from build123d import *

# Parameters (mm, degrees)
EXTRUDE_1_DEPTH      = 4
EXTRUDE_1_2_DEPTH    = 4
EXTRUDE_1_3_DEPTH    = 4
SKETCH_2_W           = 7
SKETCH_2_H           = 5
EXTRUDE_2_DEPTH      = 0.6
SKETCH_3_W           = 4.85
SKETCH_3_H           = 1.2
EXTRUDE_3_DEPTH      = 0.6
SKETCH_4_W           = 1
SKETCH_4_H           = 13.65
EXTRUDE_4_DEPTH      = 0.6
FILLET_1_R           = 0.5
FILLET_2_R           = 0.3
SKETCH_5_W           = 1.1
SKETCH_5_H           = 0.6
EXTRUDE_5_DEPTH      = 2
EXTRUDE_5_DEPTH_BACK = 18


with BuildPart() as part:
    # Sketch 1 → Extrude 1 (new body)
    with BuildSketch(Plane(origin=(0, 0, 0), x_dir=(1, 0, 0), z_dir=(0, 1, 0))):
        with BuildLine():
            Line((-2.2, 1.245389122), (2.2, 1.245389122))
            ThreePointArc((2.2, 1.245389122), (2.694974747, 1.040363869), (2.9, 0.545389122))
            Line((2.9, 0.545389122), (2.9, -1.454610878))
            ThreePointArc((2.9, -1.454610878), (2.694974747, -1.949585625), (2.2, -2.154610878))
            Line((2.2, -2.154610878), (-2.2, -2.154610878))
            ThreePointArc((-2.2, -2.154610878), (-2.694974747, -1.949585625), (-2.9, -1.454610878))
            Line((-2.9, -1.454610878), (-2.9, 0.545389122))
            ThreePointArc((-2.9, 0.545389122), (-2.694974747, 1.040363869), (-2.2, 1.245389122))
        make_face()
    extrude(amount=EXTRUDE_1_DEPTH)



with BuildPart() as body_2:
    # Sketch 1 → Extrude 1 2 (new body)
    with BuildSketch(Plane(origin=(0, 0, 0), x_dir=(1, 0, 0), z_dir=(0, 1, 0))):
        with BuildLine():
            Line((-2.2, 7.528722779), (2.2, 7.528722779))
            ThreePointArc((2.2, 7.528722779), (2.694974747, 7.323697526), (2.9, 6.828722779))
            Line((2.9, 6.828722779), (2.9, 4.828722779))
            ThreePointArc((2.9, 4.828722779), (2.694974747, 4.333748032), (2.2, 4.128722779))
            Line((2.2, 4.128722779), (-2.2, 4.128722779))
            ThreePointArc((-2.2, 4.128722779), (-2.694974747, 4.333748032), (-2.9, 4.828722779))
            Line((-2.9, 4.828722779), (-2.9, 6.828722779))
            ThreePointArc((-2.9, 6.828722779), (-2.694974747, 7.323697526), (-2.2, 7.528722779))
        make_face()
    extrude(amount=EXTRUDE_1_2_DEPTH)


with BuildPart() as body_3:
    # Sketch 1 → Extrude 1 3 (new body)
    with BuildSketch(Plane(origin=(0, 0, 0), x_dir=(1, 0, 0), z_dir=(0, 1, 0))):
        with BuildLine():
            Line((-2.2, 13.775919566), (2.2, 13.775919566))
            ThreePointArc((2.2, 13.775919566), (2.694974747, 13.570894313), (2.9, 13.075919566))
            Line((2.9, 13.075919566), (2.9, 11.075919566))
            ThreePointArc((2.9, 11.075919566), (2.694974747, 10.580944819), (2.2, 10.375919566))
            Line((2.2, 10.375919566), (-2.2, 10.375919566))
            ThreePointArc((-2.2, 10.375919566), (-2.694974747, 10.580944819), (-2.9, 11.075919566))
            Line((-2.9, 11.075919566), (-2.9, 13.075919566))
            ThreePointArc((-2.9, 13.075919566), (-2.694974747, 13.570894313), (-2.2, 13.775919566))
        make_face()
    extrude(amount=EXTRUDE_1_3_DEPTH)


with BuildPart() as part_1:
    add(part.part)

    add(body_2.part)  # Extrude 2 merges body 2

    add(body_3.part)  # Extrude 2 merges body 3
    # Sketch 2 → Extrude 2 (add)
    with BuildSketch(Plane(origin=(0, 4, 0), x_dir=(1, 0, 0), z_dir=(0, 1, 0))):
        with Locations((0.036699987, 12.063062551)):
            Rectangle(SKETCH_2_W, SKETCH_2_H)
        with Locations((0.036699987, 5.863062551)):
            Rectangle(SKETCH_2_W, SKETCH_2_H)
        with Locations((0.036699987, -0.386937449)):
            Rectangle(SKETCH_2_W, SKETCH_2_H)
    extrude(amount=-EXTRUDE_2_DEPTH)

    # Sketch 3 → Extrude 3 (add)
    with BuildSketch(Plane(origin=(0, 4, 0), x_dir=(1, 0, 0), z_dir=(0, 1, 0))):
        with Locations((5.961699987, 12.063062551)):
            Rectangle(SKETCH_3_W, SKETCH_3_H)
        with Locations((5.961699987, 5.863062551)):
            Rectangle(SKETCH_3_W, SKETCH_3_H)
        with Locations((5.961699987, -0.386937449)):
            Rectangle(SKETCH_3_W, SKETCH_3_H)
    extrude(amount=-EXTRUDE_3_DEPTH)

    # Sketch 4 → Extrude 4 (add)
    with BuildSketch(Plane.XZ.offset(-3.4)):
        with Locations((7.886699987, -5.838062551)):
            Rectangle(SKETCH_4_W, SKETCH_4_H)
    extrude(amount=-EXTRUDE_4_DEPTH)

    # Fillet 1
    fillet_1_edges = [part_1.edges().sort_by_distance(p)[0] for p in [
        (3.536699987, 3.7, -11.463062551),
        (3.536699987, 3.7, -12.663062551),
        (3.536699987, 3.7, 0.986937449),
        (3.536699987, 3.7, -0.213062551),
        (3.536699987, 3.7, -5.263062551),
        (3.536699987, 3.7, -6.463062551),
    ]]
    fillet(fillet_1_edges, radius=FILLET_1_R)

    # Fillet 2
    fillet_2_edges = [part_1.edges().sort_by_distance(p)[0] for p in [
        (-2.9, 0, 0.454610878),
        (-2.694974747, 0, -1.040363869),
        (-2.694974747, 0, -13.570894313),
        (-2.9, 0, -12.075919566),
        (-2.694974747, 0, -10.580944819),
        (0, 0, -10.375919566),
        (2.694974747, 0, -10.580944819),
        (2.9, 0, -12.075919566),
        (2.694974747, 0, -13.570894313),
        (0, 0, -13.775919566),
        (0, 0, -1.245389122),
        (2.694974747, 0, -1.040363869),
        (2.9, 0, 0.454610878),
        (2.694974747, 0, 1.949585625),
        (-2.694974747, 0, -7.323697526),
        (-2.9, 0, -5.828722779),
        (-2.694974747, 0, -4.333748032),
        (0, 0, -4.128722779),
        (2.694974747, 0, -4.333748032),
        (2.9, 0, -5.828722779),
        (0, 0, 2.154610878),
        (2.694974747, 0, -7.323697526),
        (0, 0, -7.528722779),
        (-2.694974747, 0, 1.949585625),
    ]]
    fillet(fillet_2_edges, radius=FILLET_2_R)

    # Sketch 5 → Extrude 5 (add, two sides)
    with BuildSketch(Plane(origin=(0, 0, -12.663062551), x_dir=(-1, 0, 0), z_dir=(0, 0, -1))) as extrude_5_sk:
        with Locations((-7.836699987, 3.7)):
            Rectangle(SKETCH_5_W, SKETCH_5_H)
    extrude(amount=EXTRUDE_5_DEPTH)
    extrude(extrude_5_sk.sketch, amount=-EXTRUDE_5_DEPTH_BACK)


solid = part_1.part
Verification items for the finished model (mm, model axes). A direction names the side the tool comes from. Coordinates: 2 decimals unless noted, no trailing zeros. Order: outer loops, then holes, each group sorted by start corner. A loop starts at its lowest first (then second) coordinate and runs counter-clockwise, first axis right, second up. Notation, with made-up numbers: M 36.25,-6 L 78.25,-6 A31 cw 78.25,22 Z; hole C 8.25,49 d1. An arc over 180 degrees is marked long. One line per item, written item: value. Start each with the question number.
Item 1: Gauge pin test, flat ends, axial feed: pin 1 (2 mm diameter, centred on x = 4.5, z = -9, fed in from +Y); pin 2 (2 mm diameter, centred on y = 2, z = -5.5, fed in from -X); pin 3 (2 mm diameter, centred on y = 2.5, z = -12.5, fed in from +X); pin 4 (0.5 mm diameter, centred on x = -1.5, y = 3.5, fed in from +Z). Record the tip position at first contact, or that the pin passes through.
Item 2: Sectioned sample at B-B (y = 3.15). Enter the section's corners in (x, z), then the cut area to 3 significant figures.
Item 3: Mould release check, pull along Z, two halves, no side actions. Record for faces 1 (the flat face through (0, 2, -1.245)), 2 (the flat face through (0, 0, 0)), 3 (the flat face through (0, 2, -13.776)), 4 (the flat face through (0, 2, 2.155)): released by +Z, released by -Z, zero draft, split by the parting line, or undercut.
Item 4: Sectioned sample at C-C (z = -1.5). Enter the section's corners in (x, y), then the cut area to 3 significant figures.
Item 5: Sectioned sample at D-D (z = 0.5). Enter the section's corners in (x, y), then the cut area to 3 significant figures.
Item 6: Sectioned sample at A-A (x = -1.75). Count the separate pieces of the cut face and the enclosed holes in it, then the cut area to 3 significant figures.
Item 7: Scan lines: probe 1 along Z at (x, y) = (-1.75, 1.95); probe 2 along Z at (x, y) = (7, 3.6); probe 3 along Y at (x, z) = (7.75, -2.5). Record each from-to range of solid material in increasing order.
Item 8: Access from +Z, -Z, +X, -X, +Y, -Y to the whole of each face (thin tool, end or side, straight path). Record for faces 5 (the flat face through (0, 2, -7.529)), 6 (the flat face through (-2.9, 2, 0)), 7 (the flat face through (3, 4, -7)), 8 (the flat face through (2.9, 2, -12)).
Conclusion:
1. pin 1: passes through
1. pin 2: stops at x = -2.9
1. pin 3: stops at x = 8.39
1. pin 4: stops at z = 2.89
2. outline: M -2.9,-13.08 A0.7 ccw -2.2,-13.78 L 2.2,-13.78 A0.7 ccw 2.9,-13.08 L 2.9,-11.08 A0.7 ccw 2.2,-10.38 L -2.2,-10.38 A0.7 ccw -2.9,-11.08 Z; M -2.9,-6.83 A0.7 ccw -2.2,-7.53 L 2.2,-7.53 A0.7 ccw 2.9,-6.83 L 2.9,-4.83 A0.7 ccw 2.2,-4.13 L -2.2,-4.13 A0.7 ccw -2.9,-4.83 Z; M -2.9,-0.55 A0.7 ccw -2.2,-1.25 L 2.2,-1.25 A0.7 ccw 2.9,-0.55 L 2.9,1.45 A0.7 ccw 2.2,2.15 L -2.2,2.15 A0.7 ccw -2.9,1.45 Z
2. area: 57.9 mm^2
3. face 1: undercut
3. face 2: zero draft
3. face 3: released by -Z
3. face 4: released by +Z
4. outline: M -3.46,3.4 L 3.54,3.4 L 3.54,4 L -3.46,4 Z; M 7.29,3.4 L 8.39,3.4 L 8.39,4 L 7.29,4 Z
4. area: 4.86 mm^2
5. outline: M -3.46,3.4 L -2.9,3.4 L -2.9,0.3 A0.3 ccw -2.6,0 L 2.6,0 A0.3 ccw 2.9,0.3 L 2.9,3.4 L 8.39,3.4 L 8.39,4 L -3.46,4 Z
5. area: 26.8 mm^2
6. separate pieces: 3
6. enclosed holes: 0
6. area: 43.6 mm^2
7. probe 1: z = -13.78 to -10.38, -7.53 to -4.13, -1.25 to 2.15
7. probe 2: z = -12.66 to -11.46, -6.46 to -5.26, -0.21 to 0.99
7. probe 3: y = 3.4 to 4
8. face 5: +X, -X, -Y
8. face 6: +Z, -Z, -X, -Y
8. face 7: +Z, -Z, +X, -X, +Y
8. face 8: +Z, -Z, +X, -Y
